Part model, mm, in its own coordinate system. Round coordinates to 2 decimals unless told otherwise and drop trailing zeros. Loops run counter-clockwise (first coordinate to the right, second up) from the corner with the lowest first, then second, coordinate; pieces in that order, holes last. Notation, with made-up numbers: (78, 83.25) -> (93, 83.25) arc R21 cw to (93, 90.25) -> close; hole circle Ø4 at (-15, 11). An arc over 180 degrees is marked (long way). Use a Markdown table: item, result. Add a question column.
Item 1: Cut at B-B, the plane x = -625. List the corners of the cut face in (y, z).
Item 2: Two-plate mould, pull along X, no slides. Class faces 1 (the face through (-233.506, -3.219, -487.981)), 2 (the face through (-10.53, -3.131, -609.572)), 3 (the face through (-11, -6.35, -301)), 4 (the face through (458.64, -3.22, -435.31)): pulls with the +X half, pulls with the -X half, needs draft (parallel to the pull), parting line crosses it, or undercut.
Item 3: Probe line 1 (X direction, y = -3.5, z = -175.5); line 2 (X direction, y = -2.75, z = -435); line 3 (Z direction, x = 172, y = -2.5). List the from-to ranges inside material, lowest first. Write a range as [from, to].
Item 4: Cut at A-A, the plane y = -4.25. State how many separate pieces and enclosed holes the cut face has, plus the area to 3 significant figures.
Item 5: Cut at C-C, the plane z = -76.5. List the corners of the cut face in (x, y).
```python
from build123d import *

# Parameters (mm, degrees)
F1_DEPTH        = 6.35
F2_R            = 12.7
F2_R_2          = 6.35
F3_DEPTH        = 6.351
F3_COPIES_COUNT = 4
F3_COPIES_ANGLE = 33
F6_R            = 38.1
F6_R_2          = 12.7
F7_DEPTH        = 6.351


# Not quite as in the source:
# - a pattern or mirror of a feature is missing from the dataset's text; its kind, count and spacing are read off the source's solid


with BuildPart() as f1:
    # F0 (on Front) → F1 (new body)
    with BuildSketch(Plane.XZ):
        with BuildLine():
            Line((611.4011750653, 0), (-607.7988249347, 0))
            Line((-607.7988249347, 0), (-754.3820135261, -434.6129904367))
            ThreePointArc((-754.3820135261, -434.6129904367), (-753.3868164341, -453.3515552834), (-739.7986522476, -466.2931944302))
            ThreePointArc((-739.7986522476, -466.2931944302), (0.0854683246, -609.5999981565), (739.9572217249, -466.2293582423))
            ThreePointArc((739.9572217249, -466.2293582423), (753.5060114552, -453.3692838691), (754.5955072236, -434.7208465349))
            Line((754.5955072236, -434.7208465349), (611.4011750653, 0))
        make_face()
    extrude(amount=F1_DEPTH)

    # F2 (on face) → F3 (cut, through all)
    with BuildSketch(Plane.XZ.offset(6.35)):
        with Locations((624.5911696341, -379.2573002913)):
            Circle(F2_R)
        with Locations((629.293420012, -418.017962579)):
            Circle(F2_R)
        with Locations((587.7311349843, -374.5315110857)):
            Circle(F2_R)
        with Locations((592.4333853621, -413.2921733735)):
            Circle(F2_R)
        with Locations((551.9889335366, -378.8611260422)):
            Circle(F2_R)
        with Locations((556.2118480679, -417.7637740763)):
            Circle(F2_R)
        with Locations((524.3242327175, -401.6570658257)):
            Circle(F2_R)
        with Locations((528.5470741868, -440.5597355017)):
            Circle(F2_R)
        with Locations((468.0006088828, -443.8931335302)):
            Circle(F2_R)
        with Locations((450.8607480357, -329.3439521574)):
            Circle(F2_R)
        with Locations((548.2768330983, -300.4879931354)):
            Circle(F2_R)
        Polygon((479.9608602999, -181.6468686851), (443.4298284015, -192.4678533183), (466.8752951068, -271.6184224317), (503.4063270052, -260.7974377985), align=None)
        with Locations((453.4575292546, -282.2156713453)):
            Circle(F2_R_2)
        with Locations((520.4310877351, -262.3771995177)):
            Circle(F2_R_2)
        with Locations((428.2085651104, -196.9765969155)):
            Circle(F2_R_2)
        with Locations((495.182123591, -177.138125088)):
            Circle(F2_R_2)
    f3 = extrude(amount=-F3_DEPTH, mode=Mode.SUBTRACT)

    # F3_copies: F3 ×4 about axis
    f3_copies_axis = Axis((0.085468, 0, 1371.6), (0, 1, 0))
    for i in range(1, F3_COPIES_COUNT):
        add(f3.rotate(f3_copies_axis, i * F3_COPIES_ANGLE / (F3_COPIES_COUNT - 1)), mode=Mode.SUBTRACT)

    # F6 (on face) → F7 (cut, through all)
    with BuildSketch(Plane.XZ.offset(6.35)):
        with Locations((0, -368.3)):
            Circle(F6_R)
        with Locations((-76.2, -241.3)):
            Circle(F6_R_2)
        with Locations((-25.4, -241.3)):
            Circle(F6_R_2)
        with Locations((25.4, -241.3)):
            Circle(F6_R_2)
        with Locations((76.2, -241.3)):
            Circle(F6_R_2)
    extrude(amount=-F7_DEPTH, mode=Mode.SUBTRACT)


solid = f1.part
```
A:
| question | item | result |
|---|---|---|
| 1 | outline | (-6.35, -508.43) -> (0, -508.43) -> (0, -51) -> (-6.35, -51) -> close |
| 2 | face 1 | undercut |
| 2 | face 2 | parting line crosses it |
| 2 | face 3 | needs draft |
| 2 | face 4 | undercut |
| 3 | line 1 | x = [-666.99, -501.32], [-489.02, 489.05], [501.32, 669.21] |
| 3 | line 2 | x = [-754.51, -556.34], [-531.02, -520.4], [-495.73, -442.3], [-417.19, 458.93], [477.07, 517.13], [539.97, 754.69] |
| 3 | line 3 | z = [-602.12, -520.76], [-495.44, -481.04], [-457.17, -327.87], [-244.94, 0] |
| 4 | separate pieces | 1 |
| 4 | enclosed holes | 69 |
| 4 | area | 739,000 mm^2 |
| 5 | outline | (-633.6, -6.35) -> (636.6, -6.35) -> (636.6, 0) -> (-633.6, 0) -> close |
